CAD build for the part. Positions are in the model's coordinates, mm. A direction names the side the tool comes from. Give positions to 0.01 mm unless a question says otherwise; leave off trailing zeros. Loops run counter-clockwise (first coordinate to the right, second up) from the corner with the lowest first, then second, coordinate; pieces in that order, holes last. Notation, with made-up numbers: M 14,42 L 34,42 A34 cw 34,72 Z; hole C 32.25,-22 d11. An arc over 180 degrees is marked long. One line per question, with ' | ' between items.
Solid Edge part; units mm, degrees
sketch "Sketch1" plane through (0, 0, 0) normal (0, 0, 1) x (1, 0, 0)
  line L0 (-37.5, -10) -> (-10, -10)
  line L1 (-10, -10) -> (-10, -37.5)
  line L2 (-10, -37.5) -> (10, -37.5)
  line L3 (10, -37.5) -> (10, -10)
  line L4 (10, -10) -> (37.5, -10)
  line L5 (37.5, -10) -> (37.5, 10)
  line L6 (37.5, 10) -> (10, 10)
  line L7 (10, 10) -> (10, 37.5)
  line L8 (10, 37.5) -> (-10, 37.5)
  line L9 (-10, 37.5) -> (-10, 10)
  line L10 (-10, 10) -> (-37.5, 10)
  line L11 (-37.5, 10) -> (-37.5, -10)
extrude "Protrusion1" add sketch "Sketch1" along normal blind 7
sketch "Sketch2" plane through (0, 0, 7) normal (0, 0, 1) x (1, 0, 0)
  circle A0 centre (0, 0) radius 7.5
extrude "Protrusione_Inferiore" add sketch "Sketch2" along normal blind 2.5
sketch "Sketch3" plane through (0, 0, 9.5) normal (0, 0, 1) x (1, 0, 0)
  circle A0 centre (0, 0) radius 22.5
extrude "Protrusione_Centrale" add sketch "Sketch3" along normal blind 15
chamfer "Smusso_1" distance 5 angle 45 1 edges at (-22.5, 0, 9.5)
fillet "Rotondo_1" radius 10 12 edges at (37.5, 10, 3.5) (10, 10, 3.5) (10, 37.5, 3.5) (-10, 37.5, 3.5) (-10, 10, 3.5) (-37.5, 10, 3.5) (-37.5, -10, 3.5) (-10, -10, 3.5) (-10, -37.5, 3.5) (10, -37.5, 3.5) (10, -10, 3.5) (37.5, -10, 3.5)
sketch "Sketch4" plane through (0, 0, 7) normal (0, 0, 1) x (1, 0, 0)
  circle A0 centre (-30, 0) radius 4
extrude "Cutout1" cut sketch "Sketch4" against normal up to next
pattern_circular "Pattern1" count 4 over 360 about axis through (0, 0, 7) along (0, 0, -1) of "Cutout1"
sketch "Sketch5" plane through (0, 0, 24.5) normal (0, 0, 1) x (0, 1, 0)
  circle A0 centre (0, 0) radius 17.5
extrude "Cutout2" cut sketch "Sketch5" against normal up to vertex (10 mm away)
sketch "Sketch6" plane through (0, 0, 0) normal (0.7071, -0.7071, 0) x (0.7071, 0.7071, 0)
  line L0 (-7.5, 17) -> (7.5, 17)
  line L1 (7.5, 17) -> (7.5, 22.0033)
  line L2 (7.5, 22.0033) -> (-7.5, 22.0033)
  line L3 (-7.5, 22.0033) -> (-7.5, 17)
  dimension "D1" = 7.5
  dimension "D2" = 7.5
extrude "Scavo_collegamenti_Profile_Plane1" cut sketch "Sketch6" along normal through all
sketch "Sketch7" plane through (0, 0, 24.5) normal (0, 0, 1) x (0, 1, 0)
  line L0 (-12.5, -1.5) -> (-19.5, -1.5)
  line L1 (-19.5, -1.5) -> (-19.5, 1.5)
  line L2 (-19.5, 1.5) -> (-12.5, 1.5)
  line L3 (-12.5, 1.5) -> (-12.5, -1.5)
  dimension "D1" = 19.5
  dimension "D2" = 19.5
extrude "Scavo_per_sostegno_bobine" cut sketch "Sketch7" against normal blind 5
mirror "Mirror1" about plane through (0, 0, 0) normal (0, -1, 0) of "Scavo_per_sostegno_bobine"
hole "Foro_1" at (-19.5, 0, 24.5) direction (0, 0, -1) diameter 1.567 depth 10 thread major 2 thread length 7
mirror "Mirror2" about plane through (0, 0, 0) normal (1, 0, 0) of "Foro_1"
sketch "Sketch8" plane through (0, 0, 14.5) normal (0, 0, 1) x (0, 1, 0)
  circle A0 centre (0, 0) radius 6.5
extrude "ScavoEstrusione_5" cut sketch "Sketch8" against normal blind 4
Item 1: Saw through at C-C on y = 30. Give the cut face in (x, z), and give its area (3 significant figures).
Conclusion:
outline: M -9.68,0 L -4,0 L -4,7 L -9.68,7 Z; M 4,0 L 9.68,0 L 9.68,7 L 4,7 Z | area: 79.6 mm²
Item 2: Mould opens along Y. For faces 5 (the flat face through (-24, 10, 3)), 6 (the flat face through (-1, 1, 0)), 7 (the cylindrical face through (13.01, -12.85, 3.55)), 8 (the flat face through (14, -14, 22.003)) say: pulls with the +Y half, pulls with the -Y half, needs draft (parallel to the pull), parting line crosses it, or undercut.
Conclusion:
face 5: pulls with the +Y half | face 6: needs draft | face 7: pulls with the -Y half | face 8: undercut
Item 3: 3-axis set-ups, long thin cutter, end or side, ignore diameter. For faces 1 (the cylindrical face through (3.955, -5.158, 12.528)), 2 (the cylindrical face through (-12.85, -13.01, 3.55)), 3 (the flat face through (0, -8, 9.5)), 4 (the cylindrical face through (-33.2, -2.4, 3.5)): which of +Z, -Z, +X, -X, +Y, -Y reach the whole face in a straight line?
Conclusion:
face 1: +Z | face 2: -Z, -X, -Y | face 3: none | face 4: +Z, -Z
Item 4: Saw through at A-A on z = 20.75. Give the cut face in (x, y), and give its area (3 significant figures).
Conclusion:
outline: M -1.5,-19.5 L -1.5,-17.44 A17.5 cw -1.5,17.44 L -1.5,19.5 L 1.5,19.5 L 1.5,17.44 A17.5 cw 16.48,-5.88 L 20.3,-9.7 A22.5 ccw long 9.7,-20.3 L 5.88,-16.48 A17.5 cw 1.5,-17.44 L 1.5,-19.5 Z; hole C -19.5,0 d1.57; hole C 19.5,0 d1.57 | area: 535 mm²
Item 5: Drop flat-ended pins along their axis: P1, Ø12, axis at y = -6.5, z = 21, coming from the -X side; P2, Ø3, axis at x = -5, z = 21.5, coming from the +Y side; P3, Ø8, axis at y = -18.5, z = 15.5, coming from the +X side. Give the stop position or say it passes through.
Conclusion:
P1: x = -22.49 | P2: y = 22.23 | P3: x = 17.2
Item 6: Drill centre lines: line 1 along Z through (x, y) = (-6, -14); line 2 along Y through (x, z) = (30, 2); line 3 along Z through (x, y) = (10, -18). Where is each one in solid material? Low to high. Write a range as [from, to].
Conclusion:
line 1: [0, 7], [9.5, 14.5] | line 2: [-9.68, -4], [4, 9.68] | line 3: [0, 7], [12.59, 17], [22, 24.5]
Item 7: Saw through at B-B on x = -29. Give the cut face in (y, z), and give its area (3 significant figures).
Conclusion:
outline: M -9.89,0 L -3.87,0 L -3.87,7 L -9.89,7 Z; M 3.87,0 L 9.89,0 L 9.89,7 L 3.87,7 Z | area: 84.2 mm²
Item 8: Saw through at D-D on y = -25. Give the cut face in (x, z).
Conclusion:
outline: M -10,0 L 10,0 L 10,7 L -10,7 Z
